from build123d import *

# Parameters (mm, degrees)
EXTRUDE_1_DEPTH          = 4
CUT_EXTRUDE_1_DEPTH      = 38.06287663
CUT_EXTRUDE_1_DEPTH_BACK = 7.523724759
SKETCH_3_W               = 30
SKETCH_3_H               = 55
CUT_EXTRUDE_2_DEPTH      = 1


with BuildPart() as part:
    # 草图1 → 凸台-拉伸1 (new body)
    with BuildSketch(Plane.XY):
        with BuildLine():
            Line((0, 0), (37.06287663, 0))
            ThreePointArc((37.06287663, 0), (23.31417126, 44.123406063), (28.903445872, 90))
            Line((28.903445872, 90), (0.782681423, 90))
            ThreePointArc((0.782681423, 90), (-6.518052949, 45.060087267), (0, 0))
        make_face()
    extrude(amount=EXTRUDE_1_DEPTH)

    # 草图2 → 切除-拉伸1 (cut, two sides)
    with BuildSketch(Plane(origin=(0, 0, 0), x_dir=(0, 0, -1), z_dir=(1, 0, 0))) as cut_extrude_1_sk:
        Polygon((-4, 90), (0, 90), (0, 71.181479562), align=None)
    extrude(amount=CUT_EXTRUDE_1_DEPTH, mode=Mode.SUBTRACT)
    extrude(cut_extrude_1_sk.sketch, amount=-CUT_EXTRUDE_1_DEPTH_BACK, mode=Mode.SUBTRACT)

    # 草图3 → 切除-拉伸2 (cut, symmetric)
    with BuildSketch(Plane(origin=(0, 0, 2), x_dir=(-1, 0, 0), z_dir=(0, 0, -1))):
        with Locations((-23, 42.5)):
            Rectangle(SKETCH_3_W, SKETCH_3_H)
    extrude(amount=CUT_EXTRUDE_2_DEPTH, both=True, mode=Mode.SUBTRACT)


solid = part.part
Source: CAD feature listing. Evaluate the final solid. Frame: model axes, mm. A direction names the side the tool comes from. Round coordinates to 2 decimals unless told otherwise and drop trailing zeros. Loops run counter-clockwise (first coordinate to the right, second up) from the corner with the lowest first, then second, coordinate; pieces in that order, holes last. Notation, with made-up numbers: M 55,68 L 87,68 A14 ccw 87,88 Z; hole C 33,18.25 d1. An arc over 180 degrees is marked long. Answer as CSV lines item,"result".
Q1. Pull-direction query (Y, two-part tool) for faces 3 (the face through (10, 46, 4)), 4 (the face through (-6.51, 45.7, 1.97)), 5 (the face through (16, 70, 2)), 6 (the face through (17, 43, 3)); classes: +Y half, -Y half, draft (parallel to the pull), parting line (faces both ways), or undercut.
Verdict:
face 3,"draft"
face 4,"parting line"
face 5,"undercut"
face 6,"undercut"
Q2. Cut plane D-D (z = 1.95). Return the cut outline in (x, y).
Verdict:
outline,"M -1.99,80.36 A150 ccw 0,0 L 37.06,0 A110 cw 30.03,15 L 8,15 L 8,70 L 24.03,70 A110 cw 26.06,80.36 Z"
Q3. Contact query for flat-ended pins moving along their axis: pin 1 (10 mm diameter, centred on x = 17.5, y = 16.5, fed in from -Z); pin 2 (1 mm diameter, centred on y = 40.5, z = 2, fed in from +X); pin 3 (4 mm diameter, centred on x = 27, y = 60.5, fed in from -Z). Output: stop coordinate, or through.
Verdict:
pin 1,"stops at z = 0"
pin 2,"stops at x = 8"
pin 3,"passes through"
Q4. Line query: line 1 along Z through (x, y) = (18.5, 53); line 2 along X through (y, z) = (42.5, 2.45); line 3 along Y through (x, z) = (26, 1.05). Output: solid intervals per line, ascending.
Verdict:
line 1,"z = 0 to 1, 3 to 4"
line 2,"x = -6.52 to 8"
line 3,"y = 0 to 15"
Q5. Reachability of faces 1 (the face through (19, 15, 2)), 2 (the face through (18, 0, 2)) from +Z, -Z, +X, -X, +Y, -Y: full face, straight path, thin tool, end or side. Return the list, or none.
Verdict:
face 1,"+X"
face 2,"+Z, -Z, +X, -X, -Y"
Q6. Cut plane A-A (x = 19). Return the cut outline in (y, z), plus the area to 3 significant figures.
Verdict:
outline,"M 0,0 L 71.18,0 L 90,4 L 0,4 Z; hole M 15,1 L 70,1 L 70,3 L 15,3 Z"
area,"212 mm^2"
Q7. Cut plane C-C (x = 5). Return the cut outline in (y, z).
Verdict:
outline,"M 0,0 L 71.18,0 L 90,4 L 0,4 Z"
Q8. Cut plane B-B (y = 61.5). Return the cut outline in (x, z).
Verdict:
outline,"M -5.47,0 L 23.12,0 L 23.12,1 L 8,1 L 8,3 L 23.12,3 L 23.12,4 L -5.47,4 Z"
